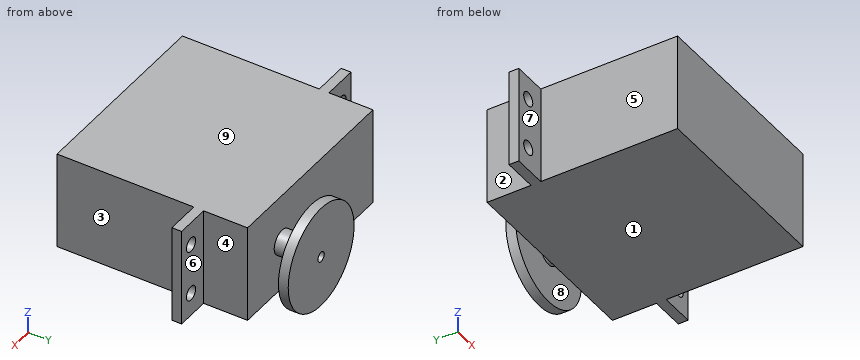
```python
from build123d import *

# Parameters (mm, degrees)
SKETCH1_W           = 40
SKETCH1_H           = 20
BOSS_EXTRUDE1_DEPTH = 39
SKETCH2_W           = 20
SKETCH2_H           = 2
BOSS_EXTRUDE2_DEPTH = 7
SKETCH3_W           = 20
SKETCH3_H           = 2
BOSS_EXTRUDE3_DEPTH = 7
SKETCH4_R           = 1.45
CUT_EXTRUDE1_DEPTH  = 31
SKETCH5_R           = 2.5
BOSS_EXTRUDE4_DEPTH = 6
SKETCH6_R           = 10.5
BOSS_EXTRUDE5_DEPTH = 2
SKETCH7_R           = 1
CUT_EXTRUDE3_DEPTH  = 6


with BuildPart() as part:
    # Sketch1 → Boss-Extrude1 (new body)
    with BuildSketch(Plane(origin=(0, 0, 0), x_dir=(1, 0, 0), z_dir=(0, 1, 0))):
        Rectangle(SKETCH1_W, SKETCH1_H)
    extrude(amount=BOSS_EXTRUDE1_DEPTH)

    # Sketch2 → Boss-Extrude2 (add)
    with BuildSketch(Plane(origin=(20, 0, 0), x_dir=(0, 0, -1), z_dir=(1, 0, 0))):
        with Locations((0, 29)):
            Rectangle(SKETCH2_W, SKETCH2_H)
    extrude(amount=BOSS_EXTRUDE2_DEPTH)

    # Sketch3 → Boss-Extrude3 (add)
    with BuildSketch(Plane.ZY.offset(20)):
        with Locations((0, 29)):
            Rectangle(SKETCH3_W, SKETCH3_H)
    extrude(amount=BOSS_EXTRUDE3_DEPTH)

    # Sketch4 → Cut-Extrude1 (cut, through all)
    with BuildSketch(Plane(origin=(0, 30, 0), x_dir=(1, 0, 0), z_dir=(0, 1, 0))):
        with Locations((24, 5.25)):
            Circle(SKETCH4_R)
        with Locations((24, -5.25)):
            Circle(SKETCH4_R)
        with Locations((-24, 5.25)):
            Circle(SKETCH4_R)
        with Locations((-24, -5.25)):
            Circle(SKETCH4_R)
    extrude(amount=-CUT_EXTRUDE1_DEPTH, mode=Mode.SUBTRACT)

    # Sketch5 → Boss-Extrude4 (add)
    with BuildSketch(Plane(origin=(0, 39, 0), x_dir=(1, 0, 0), z_dir=(0, 1, 0))):
        with Locations((9, 0)):
            Circle(SKETCH5_R)
    extrude(amount=BOSS_EXTRUDE4_DEPTH)

    # Sketch6 → Boss-Extrude5 (add)
    with BuildSketch(Plane(origin=(0, 45, 0), x_dir=(1, 0, 0), z_dir=(0, 1, 0))):
        with Locations((9, 0)):
            Circle(SKETCH6_R)
    extrude(amount=BOSS_EXTRUDE5_DEPTH)

    # Sketch7 → Cut-Extrude3 (cut)
    with BuildSketch(Plane(origin=(0, 47, 0), x_dir=(1, 0, 0), z_dir=(0, 1, 0))):
        with Locations((9, 0)):
            Circle(SKETCH7_R)
    extrude(amount=-CUT_EXTRUDE3_DEPTH, mode=Mode.SUBTRACT)


solid = part.part
```
Verification items for the finished model (mm, model axes). Face numbers are marked on the shaded views. A direction names the side the tool comes from. Give positions to 0.01 mm unless a question says otherwise; leave off trailing zeros. Loops run counter-clockwise (first coordinate to the right, second up) from the corner with the lowest first, then second, coordinate; pieces in that order, holes last. Notation, with made-up numbers: M -28,33.25 L 21,33.25 A12 cw 21,40.25 Z; hole C 4.25,67.25 d6. An arc over 180 degrees is marked long. One line per question, with ' | ' between items.
Item 1: Tool access check on the marked faces 1, 2, 3, 4 and 5. Record the directions out of +Z, -Z, +X, -X, +Y, -Y that give a thin tool (end or side, any length) a straight path to the whole face; none if there is none.
Completed:
face 1: -Z, +X, -X, -Y | face 2: +Z, -Z, -X, +Y | face 3: +Z, -Z, +X, -Y | face 4: +Z, -Z, +X, +Y | face 5: +Z, -Z, -X, -Y
Item 2: Section check D-D, the plane z = 5.25. Record the cut outline in (x, y), plus the area to 3 significant figures.
Completed:
outline: M -27,28 L -25.45,28 L -25.45,30 L -27,30 Z; M -22.55,28 L -20,28 L -20,0 L 20,0 L 20,28 L 22.55,28 L 22.55,30 L 20,30 L 20,39 L -20,39 L -20,30 L -22.55,30 Z; M -0.09,45 L 18.09,45 L 18.09,47 L -0.09,47 Z; M 25.45,28 L 27,28 L 27,30 L 25.45,30 Z | area: 1,610 mm^2
Item 3: Section check B-B, the plane z = 9. Record the cut outline in (x, y).
Completed:
outline: M -27,28 L -20,28 L -20,0 L 20,0 L 20,28 L 27,28 L 27,30 L 20,30 L 20,39 L -20,39 L -20,30 L -27,30 Z; M 3.59,45 L 14.41,45 L 14.41,47 L 3.59,47 Z
Item 4: Section check A-A, the plane x = -24. Record the cut outline in (y, z).
Completed:
outline: M 28,-10 L 30,-10 L 30,-6.7 L 28,-6.7 Z; M 28,-3.8 L 30,-3.8 L 30,3.8 L 28,3.8 Z; M 28,6.7 L 30,6.7 L 30,10 L 28,10 Z
Item 5: Draft check along Y on the marked faces 6, 7, 8 and 9. Enter one of: +Y half, -Y half, draft (parallel to the pull), parting line (faces both ways), or undercut.
Completed:
face 6: +Y half | face 7: -Y half | face 8: undercut | face 9: draft
Item 6: Section check C-C, the plane y = 43. Record the cut outline in (x, z).
Completed:
outline: C 9,0 d5; hole C 9,0 d2
Item 7: Thickness scan on line 1 (X direction, y = 29.25, z = -5.25); line 2 (Z direction, x = 24, y = 28.5); line 3 (Y direction, x = 17, z = -4). Record the ranges inside material, lowest first. Write a range as [from, to].
Completed:
line 1: x = [-27, -25.45], [-22.55, 22.55], [25.45, 27] | line 2: z = [-10, -6.7], [-3.8, 3.8], [6.7, 10] | line 3: y = [0, 39], [45, 47]
Item 8: Depth check by flat-ended pin: P1, Ø7.5, axis at x = 23, z = 3, coming from the +Y side; P2, Ø2, axis at x = 24, z = 2, coming from the -Y side; P3, Ø19.5, axis at x = -7.5, y = 15, coming from the -Z side; P4, Ø1.7, axis at x = 24, z = 5.25, coming from the -Y side (1 decimal). Enter the tip coordinate at first touch or a pass-through.
Completed:
P1: stops at y = 39 | P2: stops at y = 28 | P3: stops at z = -10 | P4: passes through
